from build123d import *

# Parameters (mm, degrees)
F4_DEPTH = 3
F1_R     = 2
F5_DEPTH = 1.5
F2_R     = 1.1
F6_DEPTH = 3
F3_W     = 33
F3_H     = 3
F7_DEPTH = 19
F9_R     = 0.5
F10_R    = 0.5


with BuildPart() as f4:
    # F0 (on Front) → F4 (new body)
    with BuildSketch(Plane.XZ):
        with BuildLine():
            Line((13.5, 8.5), (-13.5, 8.5))
            ThreePointArc((-13.5, 8.5), (-15.6213203436, 7.6213203436), (-16.5, 5.5))
            Line((-16.5, 5.5), (-16.5, 0))
            Line((-16.5, 0), (16.5, 0))
            Line((16.5, 0), (16.5, 5.5))
            ThreePointArc((16.5, 5.5), (15.6213203436, 7.6213203436), (13.5, 8.5))
        make_face()
    extrude(amount=-F4_DEPTH)

    # F1 (on Front) → F5 (cut)
    with BuildSketch(Plane.XZ):
        with Locations((-12, 5.5)):
            Circle(F1_R)
        with Locations((-4, 5.5)):
            Circle(F1_R)
        with Locations((4, 5.5)):
            Circle(F1_R)
        with Locations((12, 5.5)):
            Circle(F1_R)
    extrude(amount=-F5_DEPTH, mode=Mode.SUBTRACT)

    # F2 (on Front) → F6 (cut)
    with BuildSketch(Plane.XZ):
        with Locations((-12.0200179517, 5.5340062827)):
            Circle(F2_R)
        with Locations((-4.0200179517, 5.5340062827)):
            Circle(F2_R)
        with Locations((3.9799820483, 5.5340062827)):
            Circle(F2_R)
        with Locations((11.9799820483, 5.5340062827)):
            Circle(F2_R)
    extrude(amount=-F6_DEPTH, mode=Mode.SUBTRACT)

    # F3 (on Front) → F7 (join)
    with BuildSketch(Plane.XZ):
        with Locations((0, 1.5)):
            Rectangle(F3_W, F3_H)
    extrude(amount=-F7_DEPTH)

    # F8: F4 across face


with BuildPart() as f4_1:
    add(f4.part)
    add(f4.part.mirror(Plane(origin=(0, 19, 1.5), x_dir=(1, 0, 0), z_dir=(0, 1, 0))))

    # F9
    f9_edges = [f4_1.edges().sort_by_distance(p)[0] for p in [
        (0, 0, 8.5),
        (0, 38, 8.5),
        (16.5, 19, 3),
        (-16.5, 19, 3),
    ]]
    fillet(f9_edges, radius=F9_R)

    # F10
    f10_edges = [f4_1.edges().sort_by_distance(p)[0] for p in [
        (-16.5, 19, 0),
        (-16.353553, 37.853553, 0),
        (-16.353553, 0.146447, 0),
        (0, 38, 0),
        (0, 0, 0),
        (16.353553, 37.853553, 0),
        (16.353553, 0.146447, 0),
        (16.5, 19, 0),
    ]]
    fillet(f10_edges, radius=F10_R)


solid = f4_1.part
Work out the finished part from the listing and answer in its coordinate system (mm). A direction names the side the tool comes from. Give positions to 0.01 mm unless a question says otherwise; leave off trailing zeros. Write each loop counter-clockwise with the first axis right and the second up, starting at its lowest first coordinate (ties: lowest second). Pieces come first, ordered by that corner, then holes.
Q1. The part is cut by section A-A on x = 1. Give the vertices of the cut face in (y, z), and give its area (3 significant figures).
Answer:
outline: (0, 0.5) arc R0.5 ccw to (0.5, 0) - (37.5, 0) arc R0.5 ccw to (38, 0.5) - (38, 8) arc R0.5 ccw to (37.5, 8.5) - (35, 8.5) - (35, 3) - (3, 3) - (3, 8.5) - (0.5, 8.5) arc R0.5 ccw to (0, 8) - close
area: 147 mm2
Q2. The part is cut by section B-B on x = -12. Give the vertices of the cut face in (y, z).
Answer:
outline: (0, 0.5) arc R0.5 ccw to (0.5, 0) - (37.5, 0) arc R0.5 ccw to (38, 0.5) - (38, 3.5) - (36.5, 3.5) - (36.5, 4.43) - (35, 4.43) - (35, 3) - (3, 3) - (3, 4.43) - (1.5, 4.43) - (1.5, 3.5) - (0, 3.5) - close; (0, 7.5) - (1.5, 7.5) - (1.5, 6.63) - (3, 6.63) - (3, 8.5) - (0.5, 8.5) arc R0.5 ccw to (0, 8) - close; (35, 6.63) - (36.5, 6.63) - (36.5, 7.5) - (38, 7.5) - (38, 8) arc R0.5 ccw to (37.5, 8.5) - (35, 8.5) - close
Q3. Given pin 1 (1.3 mm diameter, centred on x = 3.98, z = 5.53, fed in from +Y); pin 2 (2 mm diameter, centred on x = 4, y = 26, fed in from +Z); pin 3 (2.5 mm diameter, centred on x = 4, z = 5.5, fed in from -Y); pin 4 (2.5 mm diameter, centred on x = -12.02, z = 5.53, fed in from +Y), each flat-ended and moving along its own axis, determine where each tip first touches the part or whether it passes through.
Answer:
pin 1: passes through
pin 2: stops at z = 3
pin 3: stops at y = 1.5
pin 4: stops at y = 36.5
Q4. The part is cut by section C-C on y = 9.5. Give the vertices of the cut face in (x, z).
Answer:
outline: (-16.5, 0.5) arc R0.5 ccw to (-16, 0) - (16, 0) arc R0.5 ccw to (16.5, 0.5) - (16.5, 2.5) arc R0.5 ccw to (16, 3) - (-16, 3) arc R0.5 ccw to (-16.5, 2.5) - close
Q5. A tool of negligible diameter and unlimited length cuts with its end or side. For faces 1 (the face through (-11.1, 1.5, 4.6)), 2 (the face through (0, 19, 3)), 3 (the face through (-11.1, 36.5, 4.6)), from which of +Z, -Z, +X, -X, +Y, -Y can it reach the whole face along a straight path? Write none if from no direction.
Answer:
face 1: -Y
face 2: +Z, +X, -X
face 3: +Y
Q6. Straight lines are drawn through the part: L1, parallel to Y at x = 6.5, z = 8; L2, parallel to Z at x = -4, y = 37; L3, parallel to Z at x = -15, y = 8.5. For each, find the intervals that lie inside material, in ascending order.
Answer:
L1: y = 0 to 3, 35 to 38
L2: z = 0 to 3.5, 7.5 to 8.5
L3: z = 0 to 3
Q7. For a pull along X with two mould halves and no side action, classify faces 4 (the face through (-15.6, 36.27, 7.64)), 5 (the face through (0, 3, 6)), 6 (the face through (11.11, 35.76, 4.86)) as released by +X, released by -X, zero draft, split by the parting line, or undercut.
Answer:
face 4: released by -X
face 5: zero draft
face 6: undercut
Q8. The part is cut by section D-D on y = 2.5. Give the vertices of the cut face in (x, z).
Answer:
outline: (-16.5, 0.5) arc R0.5 ccw to (-16, 0) - (16, 0) arc R0.5 ccw to (16.5, 0.5) - (16.5, 5.5) arc R3 ccw to (13.5, 8.5) - (-13.5, 8.5) arc R3 ccw to (-16.5, 5.5) - close; hole circle Ø2.2 at (-12.02, 5.53); hole circle Ø2.2 at (-4.02, 5.53); hole circle Ø2.2 at (3.98, 5.53); hole circle Ø2.2 at (11.98, 5.53)
